Design review of the part shown in the three views and the two pictorial views. Dimensions are in mm from the part's minimum x, y and z. Give positions to 0.01 mm unless a question says otherwise; leave off trailing zeros. Write each loop counter-clockwise with the first axis right and the second up, starting at its lowest first coordinate (ties: lowest second). Pieces come first, ordered by that corner, then holes. Notation, with made-up numbers: M 81.5,27 L 135.5,27 A22 ccw 135.5,48 Z; hole C 46,-32 d5. An arc over 180 degrees is marked long. Write item = value, one per line.
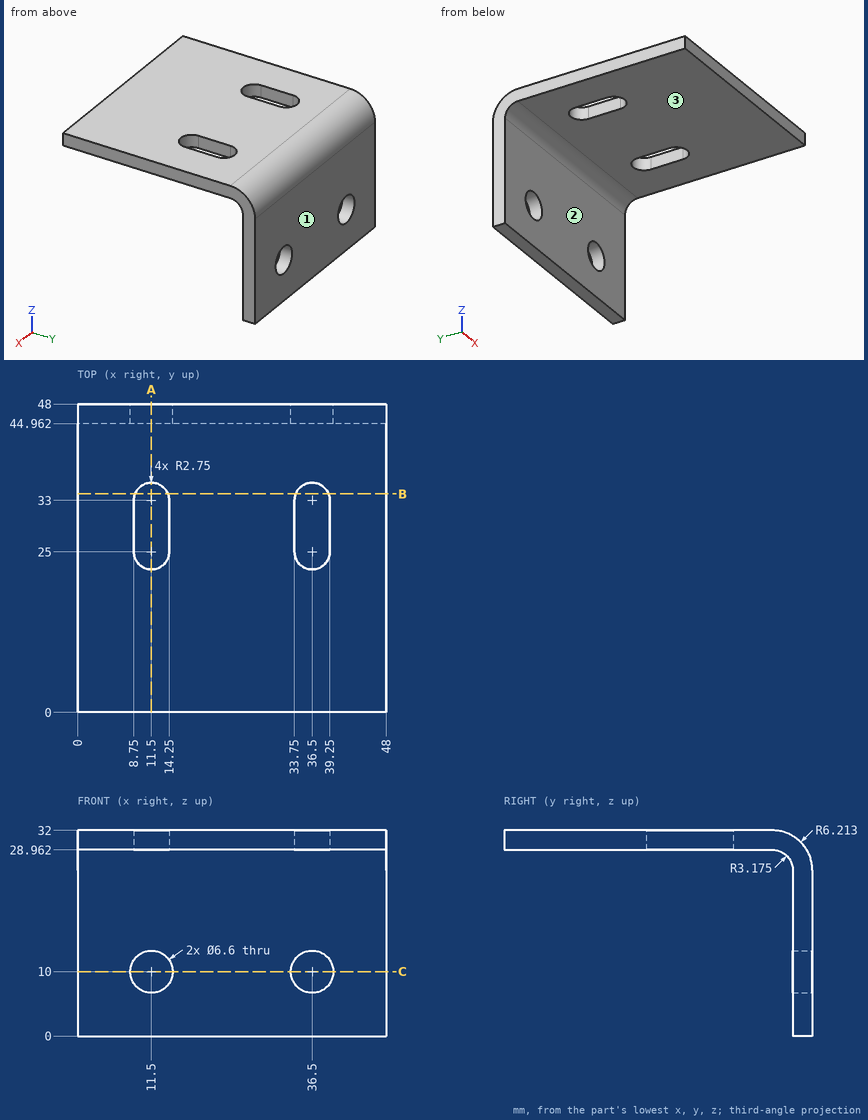
1. We need section C-C, the plane z = 10. Write out the cut boundary in (x, y), then the cut area to 3 significant figures.
Responses:
outline = M 0,44.96 L 8.2,44.96 L 8.2,48 L 0,48 Z; M 14.8,44.96 L 33.2,44.96 L 33.2,48 L 14.8,48 Z; M 39.8,44.96 L 48,44.96 L 48,48 L 39.8,48 Z
area = 106 mm2
2. We need section A-A, the plane x = 11.5. Count the separate pieces of the cut face and the enclosed holes in it, then the cut area to 3 significant figures.
Responses:
separate_pieces = 3
enclosed_holes = 0
area = 167 mm2
3. Insertion check: P1, Ø21, axis at x = 20, y = 12.5, coming from the -Z side; P2, Ø4, axis at x = 41, y = 40.5, coming from the -Z side; P3, Ø5.5, axis at x = 36.5, z = 10, coming from the -Y side; P4, Ø4, axis at x = 21, z = 14, coming from the -Y side. Each pin has a flat end and moves straight along its axis. Give the tip position at first contact, or say it passes through.
Responses:
P1 = 28.96
P2 = 28.88
P3 = through
P4 = 44.96
4. The part is to be moulded in two halves that separate along Y. For the marked faces 1, 2 and 3, say which applies: +Y half, -Y half, draft (parallel to the pull), parting line (faces both ways), or undercut.
Responses:
face_1 = +Y half
face_2 = -Y half
face_3 = draft
5. For line 1 along X through (y, z) = (45.85, 10); line 2 along Y through (x, z) = (19, 16); line 3 along Z through (x, y) = (36, 46), list the stretches that pass through material, from the lowest coordinate up. Write a range as from..to.
Responses:
line_1 = 0..8.2, 14.8..33.2, 39.8..48
line_2 = 44.96..48
line_3 = 0..6.74, 13.26..30.35
6. We need section B-B, the plane y = 34. Write out the cut boundary in (x, z), then the cut area to 3 significant figures.
Responses:
outline = M 0,28.96 L 8.94,28.96 L 8.94,32 L 0,32 Z; M 14.06,28.96 L 33.94,28.96 L 33.94,32 L 14.06,32 Z; M 39.06,28.96 L 48,28.96 L 48,32 L 39.06,32 Z
area = 115 mm2
